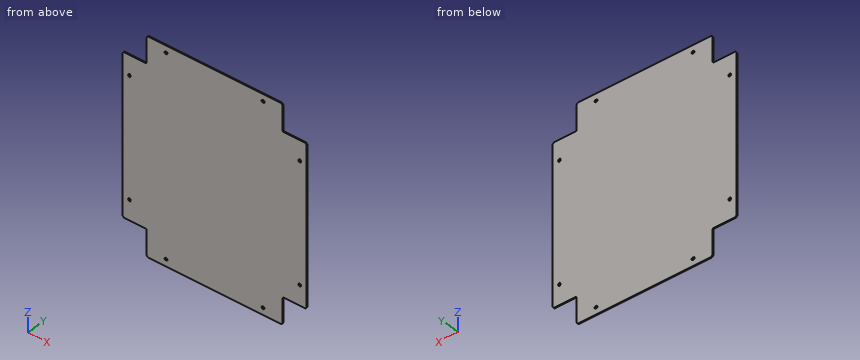
from build123d import *

# Parameters (mm, degrees)
SM_BASE_FLANGE_1_DEPTH = 1.5
CUT_EXTRUDE_1_DEPTH    = 215.212814743
FILLET_1_R             = 3.2
FILLET_3_R             = 2
CUT_EXTRUDE_2_DEPTH    = 10


# Sheet-metal steps are written as plain solids
with BuildPart() as part:
    # Sketch 1 → Базовая кромка1 (new body)
    with BuildSketch(Plane(origin=(0, 0, 0), x_dir=(1, 0, 0), z_dir=(0, 1, 0))):
        with BuildLine():
            Line((-112.2, -160.2), (112.2, -160.2))
            ThreePointArc((112.2, -160.2), (133.413203436, -151.413203436), (142.2, -130.2))
            Line((142.2, -130.2), (142.2, 130.2))
            ThreePointArc((142.2, 130.2), (133.413203436, 151.413203436), (112.2, 160.2))
            Line((112.2, 160.2), (-112.2, 160.2))
            ThreePointArc((-112.2, 160.2), (-133.413203436, 151.413203436), (-142.2, 130.2))
            Line((-142.2, 130.2), (-142.2, -130.2))
            ThreePointArc((-142.2, -130.2), (-133.413203436, -151.413203436), (-112.2, -160.2))
        make_face()
    extrude(amount=-SM_BASE_FLANGE_1_DEPTH)

    # Sketch 2 → Вырез-Вытянуть1 (cut, through all)
    with BuildSketch(Plane.XZ.offset(1.5)):
        with BuildLine():
            Line((105, 120), (142.2, 120))
            Line((142.2, 120), (142.2, 130.2))
            ThreePointArc((142.2, 130.2), (133.413203436, 151.413203436), (112.2, 160.2))
            Line((112.2, 160.2), (105, 160.2))
            Line((105, 160.2), (105, 120))
        make_face()
        with BuildLine():
            Line((142.2, -130.2), (142.2, -120))
            Line((142.2, -120), (105, -120))
            Line((105, -120), (105, -160.2))
            Line((105, -160.2), (112.2, -160.2))
            ThreePointArc((112.2, -160.2), (133.413203436, -151.413203436), (142.2, -130.2))
        make_face()
        with BuildLine():
            Line((-112.2, -160.2), (-105, -160.2))
            Line((-105, -160.2), (-105, -120))
            Line((-105, -120), (-142.2, -120))
            Line((-142.2, -120), (-142.2, -130.2))
            ThreePointArc((-142.2, -130.2), (-133.413203436, -151.413203436), (-112.2, -160.2))
        make_face()
        with BuildLine():
            Line((-105, 120), (-105, 160.2))
            Line((-105, 160.2), (-112.2, 160.2))
            ThreePointArc((-112.2, 160.2), (-133.413203436, 151.413203436), (-142.2, 130.2))
            Line((-142.2, 130.2), (-142.2, 120))
            Line((-142.2, 120), (-105, 120))
        make_face()
    extrude(amount=-CUT_EXTRUDE_1_DEPTH, mode=Mode.SUBTRACT)

    # Скругление1
    fillet_1_edges = [part.edges().sort_by_distance(p)[0] for p in [
        (-142.2, -0.75, 120),
        (-105, -0.75, 160.2),
        (-105, -0.75, -160.2),
        (-142.2, -0.75, -120),
        (105, -0.75, -160.2),
        (142.2, -0.75, -120),
        (105, -0.75, 160.2),
        (142.2, -0.75, 120),
    ]]
    fillet(fillet_1_edges, radius=FILLET_1_R)

    # Скругление3
    fillet_3_edges = [part.edges().sort_by_distance(p)[0] for p in [
        (-105, -0.75, 120),
        (-105, -0.75, -120),
        (105, -0.75, -120),
        (105, -0.75, 120),
    ]]
    fillet(fillet_3_edges, radius=FILLET_3_R)

    # Эскиз4 → Вырез-Вытянуть2 (cut)
    with BuildSketch(Plane(origin=(0, 0, 0), x_dir=(1, 0, 0), z_dir=(0, 1, 0))):
        with BuildLine():
            Line((-133.4, -90.5), (-133.4, -89.5))
            ThreePointArc((-133.4, -89.5), (-131.6, -87.7), (-129.8, -89.5))
            Line((-129.8, -89.5), (-129.8, -90.5))
            ThreePointArc((-129.8, -90.5), (-131.6, -92.3), (-133.4, -90.5))
        make_face()
        with BuildLine():
            Line((-74.5, -151.4), (-75.5, -151.4))
            ThreePointArc((-75.5, -151.4), (-77.3, -149.6), (-75.5, -147.8))
            Line((-75.5, -147.8), (-74.5, -147.8))
            ThreePointArc((-74.5, -147.8), (-72.7, -149.6), (-74.5, -151.4))
        make_face()
        with BuildLine():
            Line((-74.5, 151.4), (-75.5, 151.4))
            ThreePointArc((-75.5, 151.4), (-77.3, 149.6), (-75.5, 147.8))
            Line((-75.5, 147.8), (-74.5, 147.8))
            ThreePointArc((-74.5, 147.8), (-72.7, 149.6), (-74.5, 151.4))
        make_face()
        with BuildLine():
            Line((-133.4, 90.5), (-133.4, 89.5))
            ThreePointArc((-133.4, 89.5), (-131.6, 87.7), (-129.8, 89.5))
            Line((-129.8, 89.5), (-129.8, 90.5))
            ThreePointArc((-129.8, 90.5), (-131.6, 92.3), (-133.4, 90.5))
        make_face()
        with BuildLine():
            Line((74.5, 151.4), (75.5, 151.4))
            ThreePointArc((75.5, 151.4), (77.3, 149.6), (75.5, 147.8))
            Line((75.5, 147.8), (74.5, 147.8))
            ThreePointArc((74.5, 147.8), (72.7, 149.6), (74.5, 151.4))
        make_face()
        with BuildLine():
            Line((133.4, 90.5), (133.4, 89.5))
            ThreePointArc((133.4, 89.5), (131.6, 87.7), (129.8, 89.5))
            Line((129.8, 89.5), (129.8, 90.5))
            ThreePointArc((129.8, 90.5), (131.6, 92.3), (133.4, 90.5))
        make_face()
        with BuildLine():
            Line((133.4, -90.5), (133.4, -89.5))
            ThreePointArc((133.4, -89.5), (131.6, -87.7), (129.8, -89.5))
            Line((129.8, -89.5), (129.8, -90.5))
            ThreePointArc((129.8, -90.5), (131.6, -92.3), (133.4, -90.5))
        make_face()
        with BuildLine():
            Line((74.5, -151.4), (75.5, -151.4))
            ThreePointArc((75.5, -151.4), (77.3, -149.6), (75.5, -147.8))
            Line((75.5, -147.8), (74.5, -147.8))
            ThreePointArc((74.5, -147.8), (72.7, -149.6), (74.5, -151.4))
        make_face()
    extrude(amount=-CUT_EXTRUDE_2_DEPTH, mode=Mode.SUBTRACT)


solid = part.part
Work out the finished part from the listing and answer in its coordinate system (mm). Give positions to 0.01 mm unless a question says otherwise; leave off trailing zeros. One line per item, written item: value. Start each with the question number.
1. Find section A-A (y = -0.7). State how many separate pieces and enclosed holes the cut face has, then the cut area to 3 significant figures.
2. Given pin 1 (0.8 mm diameter, centred on y = -1, z = 142, fed in from +X), flat-ended and moving along its own axis, determine where the tip first touches the part or whether it passes through.
3. Consider probe 1 along Z at (x, y) = (-74, -0.7); probe 2 along Z at (x, y) = (-130, -0.5); probe 3 along Z at (x, y) = (-116, -0.6). Determine where each line is inside the solid, lowest interval first.
Geometry results:
1. separate pieces: 1
1. enclosed holes: 8
1. area: 85,000 mm2
2. pin 1: x = 105
3. probe 1: -160.2 to -151.33, -147.87 to 147.87, 151.33 to 160.2
3. probe 2: -120 to -91.32, -88.68 to 88.68, 91.32 to 120
3. probe 3: -120 to 120
